CAD build for the part. Positions are in the model's coordinates, mm. A direction names the side the tool comes from. Give positions to 0.01 mm unless a question says otherwise; leave off trailing zeros. Order: outer loops, then holes, each group sorted by start corner. A loop starts at its lowest first (then second) coordinate and runs counter-clockwise, first axis right, second up. Notation, with made-up numbers: (-34.5, 82) -> (18.5, 82) arc R31 cw to (18.5, 113) -> close; hole circle Ø3 at (11, 63). An arc over 180 degrees is marked (long way). Use one line per item in the form item = value. Start each with the question number.
1) Mould opens along X. For faces 1 (the face through (0.9, 8.04, 2.86)), 2 (the face through (-7, -2.5, 0)), 3 (the face through (10, 61, 29)), 4 (the face through (-10, 15, 29)) say: pulls with the +X half, pulls with the -X half, needs draft (parallel to the pull), parting line crosses it, or undercut.
2) Drop flat-ended pins along their axis: P1, Ø15, axis at x = -3, z = 10, coming from the -Y side; P2, Ø22, axis at x = -3, y = 49.5, coming from the +Z side; P3, Ø1, axis at x = 3.5, z = -32, coming from the -Y side; P4, Ø1.6, axis at x = -5, y = 64, coming from the +Z side. Give the stop position or say it passes through.
3) Cut at B-B, the plane y = 21. Give the cut face in (x, z), and give its area (3 significant figures).
4) Cut at C-C, the plane z = 18. Give the cut face in (x, y), and give its area (3 significant figures).
5) Probe line 1 (X direction, y = 2, z = 0); line 2 (X direction, y = 64, z = 31.45); line 3 (Z direction, x = -12.5, y = 33). List the from-to ranges inside material, lowest first.
6) Cut at A-A, the plane y = 49. Give the cut face in (x, z).
7) Tool access for faces 5 (the face through (0.6, -1.5, -7.8)), 6 (the face through (0, 32, -31)), 7 (the face through (0, 15, 34)), 8 (the face through (7, 59, 29)), 9 (the face through (-2.17, 39.24, -23.96)): list every direction of +Z, -Z, +X, -X, +Y, -Y with a clear straight run to the whole face (end or side of a thin tool).
8) Cut at D-D, the plane x = -32.5. Give the cut face in (y, z).
from build123d import *

# Parameters (mm, degrees)
SKETCH1_R               = 40
BOSS_EXTRUDE1_DEPTH     = 11
SKETCH3_W               = 10
SKETCH3_H               = 7
SKETCH5_R               = 3
CUT_EXTRUDE2_DEPTH      = 6
SKETCH6_W               = 30
SKETCH6_H               = 3
BOSS_EXTRUDE2_DEPTH     = 56
SKETCH7_W               = 20
SKETCH7_H               = 8
BOSS_EXTRUDE3_DEPTH     = 10
CUT_EXTRUDE4_DEPTH      = 101.920760996
CUT_EXTRUDE4_DEPTH_BACK = 5
SKETCH9_R               = 11
FILLET2_R               = 15
SKETCH13_R              = 10
BOSS_EXTRUDE4_DEPTH     = 0.5
SKETCH14_R              = 1
BOSS_EXTRUDE5_DEPTH     = 2
SKETCH4_R               = 1.5
CUT_EXTRUDE1_DEPTH      = 80.598994969
SKETCH15_W              = 30
SKETCH15_H              = 10
BOSS_EXTRUDE6_DEPTH     = 56
FILLET3_R               = 15
SKETCH16_R              = 1
CUT_EXTRUDE5_DEPTH      = 5
SKETCH20_R              = 10
CUT_EXTRUDE8_DEPTH      = 6
SKETCH22_R              = 9.171602893
CUT_EXTRUDE9_DEPTH      = 6
SKETCH23_W              = 8.009683582
SKETCH23_H              = 20
CUT_EXTRUDE10_DEPTH     = 14


with BuildPart() as part:
    # Sketch1 → Boss-Extrude1 (new body)
    with BuildSketch(Plane(origin=(0, 0, 0), x_dir=(1, 0, 0), z_dir=(0, 1, 0))):
        with Locations(Location((0, 0, 0), (0, 0, 270))):
            Circle(SKETCH1_R)
    extrude(amount=BOSS_EXTRUDE1_DEPTH)

    # Sketch3 → Cut-Revolve1 (revolve, cut)
    with BuildSketch(Plane.XY, mode=Mode.PRIVATE) as cut_revolve1_sk:
        with Locations((-30, 3.5)):
            Rectangle(SKETCH3_W, SKETCH3_H)
    revolve(cut_revolve1_sk.sketch.rotate(Axis((0, 17.41193703, 0), (0, -1, 0)), 270), axis=Axis((0, 17.41193703, 0), (0, -1, 0)), mode=Mode.SUBTRACT)

    # Sketch5 → Cut-Extrude2 (cut)
    with BuildSketch(Plane(origin=(0, 11, 0), x_dir=(1, 0, 0), z_dir=(0, 1, 0))):
        with Locations(Location((0, 0, 0), (0, 0, 270))):
            Circle(SKETCH5_R)
    extrude(amount=-CUT_EXTRUDE2_DEPTH, mode=Mode.SUBTRACT)

    # Sketch6 → Boss-Extrude2 (add)
    with BuildSketch(Plane(origin=(0, 11, 0), x_dir=(1, 0, 0), z_dir=(0, 1, 0))):
        with Locations((0, -22.5)):
            Rectangle(SKETCH6_W, SKETCH6_H)
    extrude(amount=BOSS_EXTRUDE2_DEPTH)

    # Sketch7 → Boss-Extrude3 (add)
    with BuildSketch(Plane.XY.offset(24)):
        with Locations((0, 15)):
            Rectangle(SKETCH7_W, SKETCH7_H)
        with Locations((0, 63)):
            Rectangle(SKETCH7_W, SKETCH7_H)
    extrude(amount=BOSS_EXTRUDE3_DEPTH)

    # Sketch9 → Cut-Extrude4 (cut, two sides: drawn at the far end of the back side and taken through both)
    with BuildSketch(Plane.XY.offset(24).offset(-CUT_EXTRUDE4_DEPTH_BACK)):
        with Locations(Location((0, 49, 0), (0, 0, 114.619977329))):
            Circle(SKETCH9_R)
    extrude(amount=CUT_EXTRUDE4_DEPTH + CUT_EXTRUDE4_DEPTH_BACK, mode=Mode.SUBTRACT)

    # Fillet2
    fillet2_edges = [part.edges().sort_by_distance(p)[0] for p in [
        (15, 67, 22.5),
        (-15, 67, 22.5),
    ]]
    fillet(fillet2_edges, radius=FILLET2_R - 0.0001)  # a hair under: the kernel refuses the full size

    # Sketch13 → Boss-Extrude4 (add)
    with BuildSketch(Plane.XZ):
        with Locations(Location((0, 0, 0), (0, 0, 270))):
            Circle(SKETCH13_R)
    extrude(amount=BOSS_EXTRUDE4_DEPTH)

    # Sketch14 → Boss-Extrude5 (add)
    with BuildSketch(Plane.XZ.offset(0.5)):
        with Locations(Location((0, 7, 0), (0, 0, 270))):
            Circle(SKETCH14_R)
        with Locations(Location((0, -7, 0), (0, 0, 90))):
            Circle(SKETCH14_R)
        with Locations(Location((7.141428429, 0, 0), (0, 0, 270))):
            Circle(SKETCH14_R)
        with Locations(Location((-7.141428429, 0, 0), (0, 0, 90))):
            Circle(SKETCH14_R)
    extrude(amount=BOSS_EXTRUDE5_DEPTH)

    # Sketch4 → Cut-Extrude1 (cut, through all)
    with BuildSketch(Plane(origin=(0, 11, 0), x_dir=(1, 0, 0), z_dir=(0, 1, 0))):
        with Locations(Location((0, 0, 0), (0, 0, 270))):
            Circle(SKETCH4_R)
    extrude(amount=-CUT_EXTRUDE1_DEPTH, mode=Mode.SUBTRACT)

    # Sketch15 → Boss-Extrude6 (add)
    with BuildSketch(Plane(origin=(0, 11, 0), x_dir=(1, 0, 0), z_dir=(0, 1, 0))):
        with Locations((0, 26)):
            Rectangle(SKETCH15_W, SKETCH15_H)
    extrude(amount=BOSS_EXTRUDE6_DEPTH)

    # Fillet3
    fillet3_edges = [part.edges().sort_by_distance(p)[0] for p in [
        (-15, 67, -26),
        (15, 67, -26),
    ]]
    fillet(fillet3_edges, radius=FILLET3_R - 0.0001)  # a hair under: the kernel refuses the full size

    # Sketch16 → Cut-Extrude5 (cut)
    with BuildSketch(Plane.XY.offset(34)):
        with Locations((-5, 64)):
            Circle(SKETCH16_R)
        with Locations(Location((5, 64, 0), (0, 0, 180))):
            Circle(SKETCH16_R)
        with Locations(Location((-5, 14, 0), (0, 0, 180))):
            Circle(SKETCH16_R)
        with Locations((5, 14)):
            Circle(SKETCH16_R)
    extrude(amount=-CUT_EXTRUDE5_DEPTH, mode=Mode.SUBTRACT)

    # Sketch20 → Cut-Extrude8 (cut)
    with BuildSketch(Plane.XY.offset(-21)):
        with Locations((0, 49)):
            Circle(SKETCH20_R)
    extrude(amount=-CUT_EXTRUDE8_DEPTH, mode=Mode.SUBTRACT)

    # Sketch22 → Cut-Extrude9 (cut)
    with BuildSketch(Plane.XY.offset(-27)):
        with Locations((0, 49)):
            Circle(SKETCH22_R)
    extrude(amount=-CUT_EXTRUDE9_DEPTH, mode=Mode.SUBTRACT)

    # Sketch23 → Cut-Extrude10 (cut)
    with BuildSketch(Plane.XZ):
        with Locations((15.018156717, 0)):
            Rectangle(SKETCH23_W, SKETCH23_H)
    extrude(amount=-CUT_EXTRUDE10_DEPTH, mode=Mode.SUBTRACT)


solid = part.part
Result:
q1.face_1 = undercut
q1.face_2 = needs draft
q1.face_3 = pulls with the +X half
q1.face_4 = pulls with the -X half
q2.P1 = -2.5
q2.P2 = 34
q2.P3 = 7
q2.P4 = 29
q3.outline = (-15, -31) -> (15, -31) -> (15, -21) -> (-15, -21) -> close; (-15, 21) -> (15, 21) -> (15, 24) -> (-15, 24) -> close
q3.area = 390 mm²
q4.outline = (-35.72, 0) -> (-30.02, 0) -> (-30.02, 7) -> (-17.35, 7) -> (-17.35, 0) -> (17.35, 0) -> (17.35, 7) -> (30.02, 7) -> (30.02, 0) -> (35.72, 0) -> (35.72, 11) -> (-35.72, 11) -> close
q4.area = 609 mm²
q5.line_1 = -40 to -35, -25 to -1.5, 1.5 to 11.01, 19.02 to 25, 35 to 40
q5.line_2 = -9 to -6, -4 to 4, 6 to 9
q5.line_3 = -31 to -21, 21 to 24
q6.outline = (-15, -31) -> (-9.17, -31) -> (-9.17, -27) -> (-10, -27) -> (-10, -21) -> (-15, -21) -> close; (-15, 21) -> (-11, 21) -> (-11, 24) -> (-15, 24) -> close; (9.17, -31) -> (15, -31) -> (15, -21) -> (10, -21) -> (10, -27) -> (9.17, -27) -> close; (11, 21) -> (15, 21) -> (15, 24) -> (11, 24) -> close
q7.face_5 = -Y
q7.face_6 = -Z, +X, -X, +Y
q7.face_7 = +Z, +X, -X, +Y
q7.face_8 = +Z, +X, -X
q7.face_9 = +Z
q8.outline = (0, -23.32) -> (11, -23.32) -> (11, 23.32) -> (0, 23.32) -> (0, 12.99) -> (7, 12.99) -> (7, -12.99) -> (0, -12.99) -> close
